Geometry check sheet. Reference: the model listing, model coordinates, mm. A direction names the side the tool comes from. Round coordinates to 2 decimals unless told otherwise and drop trailing zeros. Order: outer loops, then holes, each group sorted by start corner. A loop starts at its lowest first (then second) coordinate and runs counter-clockwise, first axis right, second up. Notation, with made-up numbers: (73, 1) - (111, 1) arc R31 cw to (111, 27) - close; hole circle Ø6 at (6, -8.75). An arc over 180 degrees is marked (long way). One line per question, with ' | ' between items. Start each with the question number.
Q1. Sectioned sample at C-C, the plane x = 0. Enter the section's corners in (y, z).
Q2. Sectioned sample at A-A, the plane z = 8. Enter the section's corners in (x, y).
Q3. Sectioned sample at D-D, the plane x = 16.5. Give the number of separate pieces and of enclosed holes in the cut face, then the cut area to 3 significant figures.
Q4. Mould release check, pull along X, two halves, no side actions. Record for faces 1 (the face through (45, 0, 0)), 2 (the face through (-59.94, 2.64, 0.15)), 3 (the face through (-14, -12, -12.5)): +X half, -X half, draft (parallel to the pull), parting line (faces both ways), or undercut.
Q5. Sectioned sample at B-B, the plane y = 0. Enter the section's corners in (x, z), then the cut area to 3 significant figures.
Q6. Tool access check on faces 4 (the face through (5.98, -0.31, 0.18)), 5 (the face through (-14, -12, 12.5)). Record the directions out of +Z, -Z, +X, -X, +Y, -Y that give a thin tool (end or side, any length) a straight path to the whole face; none if there is none.
Q7. Material ranges on line 1 along Y through (x, z) = (0, -6); line 2 along X through (y, z) = (-10.5, -5.75); line 3 along X through (y, z) = (2, -7.25), recorded low to high.
Q8. Gauge pin test, flat ends, axial feed: P1, Ø7.5, axis at x = 1, z = 6, coming from the -Y side; P2, Ø1.5, axis at x = -22.5, z = 5.5, coming from the -Y side; P3, Ø4, axis at x = 46, z = -3, coming from the -Y side. Record the tip position at first contact, or that the pin passes through.
```python
from build123d import *

# Parameters (mm, degrees)
F0_R     = 60
F0_R_2   = 45
F1_DEPTH = 12.5
F2_SIZE  = 2
F3_R     = 2.5
F4_DEPTH = 12.5
F6_DEPTH = 12.5


with BuildPart() as f1:
    # F0 (on Top) → F1 (new body, symmetric)
    with BuildSketch(Plane.XY):
        Circle(F0_R)
        Circle(F0_R_2, mode=Mode.SUBTRACT)
    extrude(amount=F1_DEPTH, both=True)

    # F2
    f2_edges = [f1.edges().sort_by_distance(p)[0] for p in [
        (-60, 0, -12.5),
        (-60, 0, 12.5),
    ]]
    chamfer(f2_edges, length=F2_SIZE)

    # F3 (on Top) → F4 (join, symmetric)
    with BuildSketch(Plane.XY):
        Polygon((37.510756, 25.18704), (32.372119, 31.320056), (-37.304859, -25.020552), (-32.410452, -31.351052), align=None)
        Circle(F3_R, mode=Mode.SUBTRACT)
    extrude(amount=F4_DEPTH, both=True)

    # F5 (on face) → F6 (join, symmetric)
    with BuildSketch(Plane.XY):
        Polygon((38.118351, -24.993353), (-24.714097, -24.993353), (-31.974737, -30.857714), (32.812502, -30.857714), align=None)
    extrude(amount=F6_DEPTH, both=True)


solid = f1.part
```
Determined:
1) outline: (-60, -10.5) - (-58, -12.5) - (-45, -12.5) - (-45, 12.5) - (-58, 12.5) - (-60, 10.5) - close; (-30.86, -12.5) - (-24.99, -12.5) - (-24.99, 12.5) - (-30.86, 12.5) - close; (-5.14, -12.5) - (-2.5, -12.5) - (-2.5, 12.5) - (-5.14, 12.5) - close; (2.5, -12.5) - (5.14, -12.5) - (5.14, 12.5) - (2.5, 12.5) - close; (45, -12.5) - (58, -12.5) - (60, -10.5) - (60, 10.5) - (58, 12.5) - (45, 12.5) - close
2) outline: circle Ø120 at (0, 0); hole (-37.3, -25.02) - (32.34, 31.29) arc R45 ccw to (-32.97, -30.62) - close; hole (-32.34, -31.29) arc R45 ccw to (32.75, -30.86) - (-31.8, -30.86) - close; hole (-24.55, -24.99) - (37.42, -24.99) arc R45 ccw to (37.37, 25.07) - close; hole circle Ø5 at (0, 0); hole (32.81, 30.8) - (36.07, 26.91) arc R45 ccw to start
3) separate pieces: 4 | enclosed holes: 0 | area: 1,190 mm2
4) face 1: undercut | face 2: parting line | face 3: draft
5) outline: (-60, -10.5) - (-58, -12.5) - (-45, -12.5) - (-45, 12.5) - (-58, 12.5) - (-60, 10.5) - close; (-6.36, -12.5) - (-2.5, -12.5) - (-2.5, 12.5) - (-6.36, 12.5) - close; (2.5, -12.5) - (6.36, -12.5) - (6.36, 12.5) - (2.5, 12.5) - close; (45, -12.5) - (58, -12.5) - (60, -10.5) - (60, 10.5) - (58, 12.5) - (45, 12.5) - close | area: 935 mm2
6) face 4: +Z, -Z | face 5: +Z, +X, -X, +Y, -Y
7) line 1: y = -60 to -45, -30.86 to -24.99, -5.14 to -2.5, 2.5 to 5.14, 45 to 60 | line 2: x = -59.07 to -43.76, -19.35 to -6.62, 43.76 to 59.07 | line 3: x = -59.97 to -44.96, -3.89 to -1.5, 1.5 to 8.84, 44.96 to 59.97
8) P1: stops at y = -60 | P2: stops at y = -55.92 | P3: stops at y = -40.79
